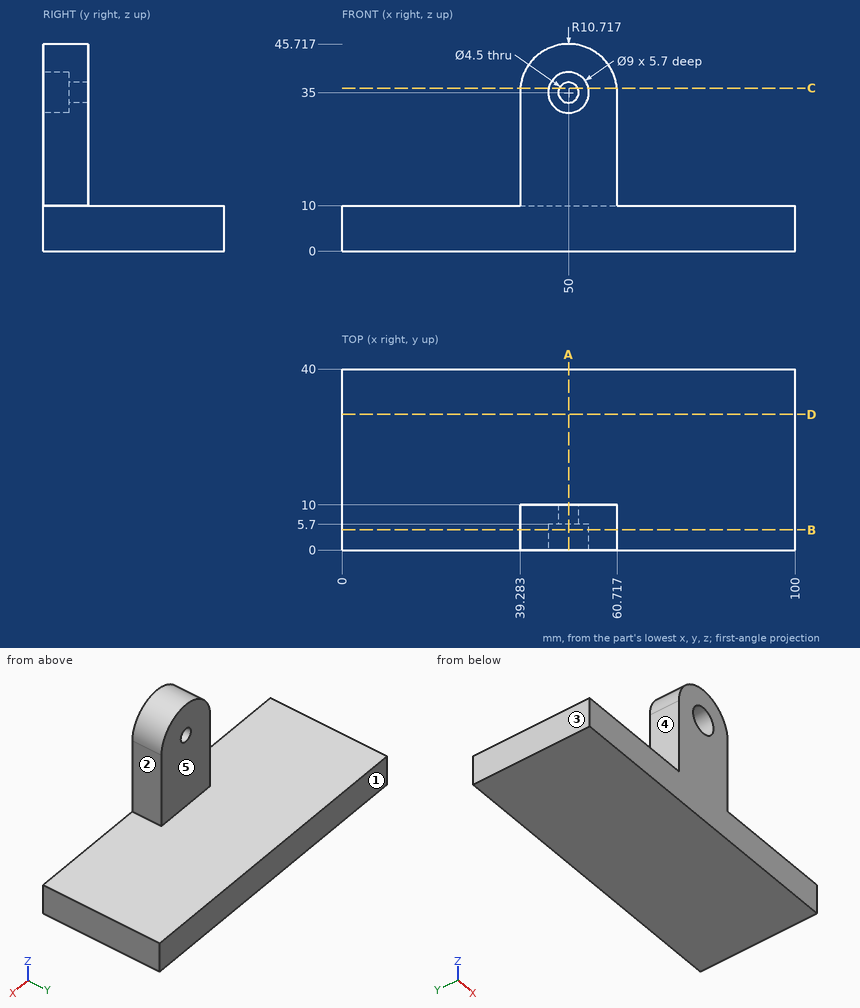
Part print with two shaded views. Sizes in mm from the minimum x, y, z corner. A direction names the side the tool comes from. Give positions to 0.01 mm unless a question says otherwise; leave off trailing zeros. Order: outer loops, then holes, each group sorted by start corner. A loop starts at its lowest first (then second) coordinate and runs counter-clockwise, first axis right, second up.
1) 3-axis set-ups, long thin cutter, end or side, ignore diameter. For the marked faces 1, 2, 3, 4 and 5: which of +Z, -Z, +X, -X, +Y, -Y reach the whole face in a straight line?
2) Saw through at C-C, the plane z = 36. Write the cut outline in (x, y).
3) Saw through at B-B, the plane y = 4.5. Write the cut outline in (x, z).
4) Saw through at D-D, the plane y = 30. Write the cut outline in (x, z), then the cut area to 3 significant figures.
5) Pin check, flat tips, straight feed: pin 1 (3 mm diameter, centred on y = 7, z = 21, fed in from +X); pin 2 (4.5 mm diameter, centred on x = 50, z = 33.5, fed in from -Y); pin 3 (7 mm diameter, centred on x = 50, z = 35, fed in from +Y). Stop position of each tip, or through.
6) Wall check: probe 1 along Z at (x, y) = (50, 1.55); probe 2 along Z at (x, y) = (50, 7); probe 3 along Y at (x, z) = (41, 21). Give the ranges that are in metal, low to high.
7) Saw through at A-A, the plane x = 50. Write the cut outline in (y, z), then the cut area to 3 significant figures.
Computed:
1. face 1: +Z, -Z, +X, -X, +Y
1. face 2: +Z, +X, +Y, -Y
1. face 3: +Z, -Z, -X, +Y, -Y
1. face 4: +Z, -X, +Y, -Y
1. face 5: +Z, +X, -X, +Y
2. outline: (39.33, 0) - (45.61, 0) - (45.61, 5.7) - (47.98, 5.7) - (47.98, 10) - (39.33, 10) - close; (52.02, 5.7) - (54.39, 5.7) - (54.39, 0) - (60.67, 0) - (60.67, 10) - (52.02, 10) - close
3. outline: (0, 0) - (100, 0) - (100, 10) - (60.72, 10) - (60.72, 35) arc R10.72 ccw to (39.28, 35) - (39.28, 10) - (0, 10) - close; hole circle Ø9 at (50, 35)
4. outline: (0, 0) - (100, 0) - (100, 10) - (0, 10) - close
4. area: 1,000 mm2
5. pin 1: stops at x = 60.72
5. pin 2: stops at y = 5.7
5. pin 3: stops at y = 10
6. probe 1: z = 0 to 30.5, 39.5 to 45.72
6. probe 2: z = 0 to 32.75, 37.25 to 45.72
6. probe 3: y = 0 to 10
7. outline: (0, 0) - (40, 0) - (40, 10) - (10, 10) - (10, 32.75) - (5.7, 32.75) - (5.7, 30.5) - (0, 30.5) - close; (0, 39.5) - (5.7, 39.5) - (5.7, 37.25) - (10, 37.25) - (10, 45.72) - (0, 45.72) - close
7. area: 687 mm2
